Can you work these out from the model? Positions are in its coordinate system, mm. Face numbers are marked on the shaded views. A direction names the side the tool comes from. Coordinates: 2 decimals unless noted, no trailing zeros. Loops run counter-clockwise (first coordinate to the right, second up) from the corner with the lowest first, then second, coordinate; pieces in that order, holes last. Notation, with made-up numbers: M 33.25,27 L 73.25,27 A30 ccw 73.25,58 Z; hole C 37.5,49.5 d9. An arc over 180 degrees is marked long. Answer as a JSON object with one key per item and string values. Group by question number.
Item 1: Suppose I cut it at C-C (z = 7). Write out the boundary of the cut face in (x, y) (3 decimals).
Item 2: Suppose I cut it at B-B (x = 12). Write out the boundary of the cut face in (y, z).
Item 3: Suppose I cut it at A-A (z = 1). Write out the boundary of the cut face in (x, y), then the cut area to 3 significant figures.
Item 4: Which directions (+Z, -Z, +X, -X, +Y, -Y) give clear straight access to the entire face, cutting with the end or side of a thin tool? Please do the marked faces 1, 2, 3, 4 and 5.
Item 5: I'm going to push flat-ended pins straight in: pin 1 Ø1.8 at (x, y) = (-4.5, 9.5) entering from -Z; pin 2 Ø2 at (y, z) = (-5.5, 4.5) entering from +X; pin 3 Ø2.5 at (x, y) = (-12.5, -0.5) entering from +Z. Where does each tip first touch, or does it pass through?
Item 6: If I drill on line 1 (X direction, y = -10, z = 7); line 2 (Y direction, x = 0, z = 3.5); line 3 (X direction, y = -9, z = 4.25), over which ranges is the centre line in solid material (lowest first)?
Item 7: We'd pull the mould along Z, two halves only. Please class the marked faces 6, 7, 8 and 9: +Z half, -Z half, draft (parallel to the pull), parting line (faces both ways), or undercut.
Item 8: Suppose I cut it at D-D (y = -0.5). Count the separate pieces of the cut face and the enclosed holes in it, then the cut area to 3 significant figures.
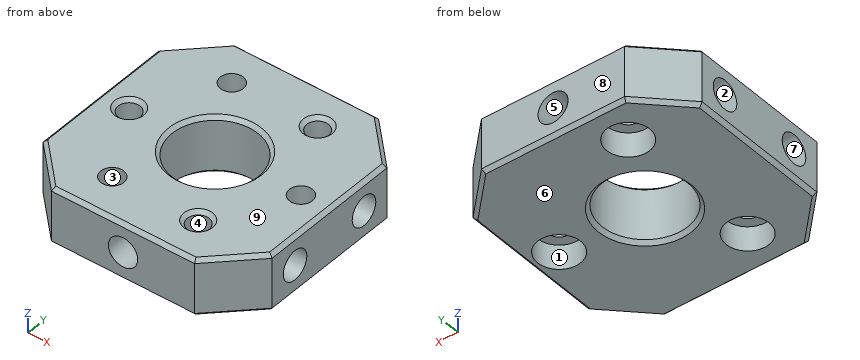
```python
from build123d import *

# Parameters (mm, degrees)
SKETCH_1_W                   = 32
SKETCH_1_H                   = 32
SKETCH_1_R                   = 6
EXTRUDE_1_DEPTH              = 8
SKETCH_2_R                   = 1.525
CUT_EXTRUDE_1_DEPTH          = 4
CHAMFER_1_SIZE               = 6
SKETCH_4_R                   = 2.1
CUT_EXTRUDE_2_DEPTH          = 4.5
SKETCH_5_R                   = 2.05
CUT_EXTRUDE_3_DEPTH          = 4.5
SKETCH_6_R                   = 2.05
CUT_EXTRUDE_4_DEPTH          = 4.5
CUT_EXTRUDE_START            = -4.5
SKETCH_7_R                   = 2.05
CUT_EXTRUDE_5_DEPTH          = 4.5
CHAMFER_2_SIZE               = 0.5
HOLE_WIZARD_M3_1_D           = 3.2
HOLE_WIZARD_M3_1_CBORE_D     = 6
HOLE_WIZARD_M3_1_CBORE_DEPTH = 3.4


with BuildPart() as part:
    # 草图1 → 凸台-拉伸1 (new body)
    with BuildSketch(Plane.XY):
        Rectangle(SKETCH_1_W, SKETCH_1_H)
        Circle(SKETCH_1_R, mode=Mode.SUBTRACT)
    extrude(amount=EXTRUDE_1_DEPTH)

    # 草图2 → 切除-拉伸1 (cut)
    with BuildSketch(Plane.XY.offset(8)):
        with Locations((-12, 0)):
            Circle(SKETCH_2_R)
        with Locations((6, 10.392304845)):
            Circle(SKETCH_2_R)
        with Locations((6, -10.392304845)):
            Circle(SKETCH_2_R)
    extrude(amount=-CUT_EXTRUDE_1_DEPTH, mode=Mode.SUBTRACT)

    # 倒角1
    chamfer_1_edges = [part.edges().sort_by_distance(p)[0] for p in [
        (16, -16, 4),
        (-16, -16, 4),
        (-16, 16, 4),
        (16, 16, 4),
    ]]
    chamfer(chamfer_1_edges, length=CHAMFER_1_SIZE)

    # 草图4 → 切除-拉伸2 (cut)
    with BuildSketch(Plane(origin=(0, 16, 0), x_dir=(1, 0, 0), z_dir=(0, 1, 0))):
        with Locations(Location((0, -4, 0), (0, 0, 270))):
            Circle(SKETCH_4_R)
    extrude(amount=-CUT_EXTRUDE_2_DEPTH, mode=Mode.SUBTRACT)

    # 草图5 → 切除-拉伸3 (cut)
    with BuildSketch(Plane.XZ.offset(16)):
        with Locations(Location((0, 4, 0), (0, 0, 270))):
            Circle(SKETCH_5_R)
    extrude(amount=-CUT_EXTRUDE_3_DEPTH, mode=Mode.SUBTRACT)

    # 草图6 → 切除-拉伸4 (cut)
    with BuildSketch(Plane(origin=(16, 0, 0), x_dir=(0, 0, -1), z_dir=(1, 0, 0))):
        with Locations((-4, 6)):
            Circle(SKETCH_6_R)
        with Locations((-4, -6)):
            Circle(SKETCH_6_R)
    extrude(amount=-CUT_EXTRUDE_4_DEPTH, mode=Mode.SUBTRACT)

    # 草图7 → 切除-拉伸5 (cut)
    with BuildSketch(Plane.ZY.offset(16).offset(CUT_EXTRUDE_START)):
        with Locations(Location((4, 6, 0), (0, 0, 180))):
            Circle(SKETCH_7_R)
        with Locations(Location((4, -6, 0), (0, 0, 180))):
            Circle(SKETCH_7_R)
    extrude(amount=CUT_EXTRUDE_5_DEPTH, mode=Mode.SUBTRACT)

    # 倒角2
    chamfer_2_edges = [part.edges().sort_by_distance(p)[0] for p in [
        (-6, 0, 0),
        (-6, 0, 8),
        (-13.525, 0, 8),
        (4.475, 10.392304845, 8),
        (4.475, -10.392304845, 8),
        (0, -16, 0),
        (0, -16, 8),
        (16, 0, 0),
        (-16, 0, 0),
        (0, 16, 0),
        (13, 13, 0),
        (-13, 13, 0),
        (13, -13, 0),
        (-13, -13, 0),
        (-16, 0, 8),
        (16, 0, 8),
        (0, 16, 8),
        (13, 13, 8),
        (-13, 13, 8),
        (13, -13, 8),
        (-13, -13, 8),
    ]]
    chamfer(chamfer_2_edges, length=CHAMFER_2_SIZE)

    # M3 六角圆柱头螺钉的柱形沉头孔1 (through all)
    with Locations(Plane(origin=(0, 0, 0), x_dir=(-1, 0, 0), z_dir=(0, 0, -1))):
        with Locations((-12, 0), (6, 10.392304845), (6, -10.392304845)):
            CounterBoreHole(HOLE_WIZARD_M3_1_D / 2, HOLE_WIZARD_M3_1_CBORE_D / 2, HOLE_WIZARD_M3_1_CBORE_DEPTH)


solid = part.part
```
From the geometry:
{
 "1": {"outline": "M -16,-10 L -10,-16 L 10,-16 L 16,-10 L 16,10 L 10,16 L -10,16 L -16,10 Z; hole C -12,0 d3.05; hole C -6,-10.392 d3.2; hole C -6,10.392 d3.2; hole C 0,0 d12; hole C 6,-10.392 d3.05; hole C 6,10.392 d3.05; hole C 12,0 d3.2"},
 "2": {"outline": "M -14,0.5 L -13.29,0 L -3,0 L -3,3.4 L -1.6,3.4 L -1.6,8 L -13.29,8 L -14,7.5 Z; M 1.6,3.4 L 3,3.4 L 3,0 L 13.29,0 L 14,0.5 L 14,7.5 L 13.29,8 L 1.6,8 Z; hole C -6,4 d4.1; hole C 6,4 d4.1"},
 "3": {"outline": "M -16,-10 L -10,-16 L 10,-16 L 16,-10 L 16,10 L 10,16 L -10,16 L -16,10 Z; hole C -6,-10.39 d6; hole C -6,10.39 d6; hole C 0,0 d12; hole C 12,0 d6", "area": "754 mm2"},
 "4": {"face 1": "-Z", "face 2": "-X", "face 3": "+Z, -Z", "face 4": "+Z", "face 5": "+Y"},
 "5": {"pin 1": "z = 3.4", "pin 2": "x = 11.5", "pin 3": "z = 7.93"},
 "6": {"line 1": "-16 to -7.55, -4.45 to 4.53, 7.47 to 16", "line 2": "-11.5 to -6, 6 to 11.5", "line 3": "-16 to -6.79, -5.21 to 5.38, 6.62 to 16"},
 "7": {"face 6": "-Z half", "face 7": "undercut", "face 8": "draft", "face 9": "+Z half"},
 "8": {"separate pieces": "3", "enclosed holes": "0", "area": "113 mm2"}
}
